The figure shows three views and two pictorial views of one solid part (mm, origin at its lowest corner). Answer the questions. A direction names the side the tool comes from. Round coordinates to 2 decimals unless told otherwise and drop trailing zeros. Order: outer loops, then holes, each group sorted by start corner. A loop starts at its lowest first (then second) coordinate and runs counter-clockwise, first axis right, second up. Notation, with made-up numbers: (58, -15) -> (101, -15) arc R19 ccw to (101, -4) -> close; hole circle Ø5 at (37, -10.5). An arc over 180 degrees is marked (long way). Answer in a Markdown table with one row per item. Add a question column.
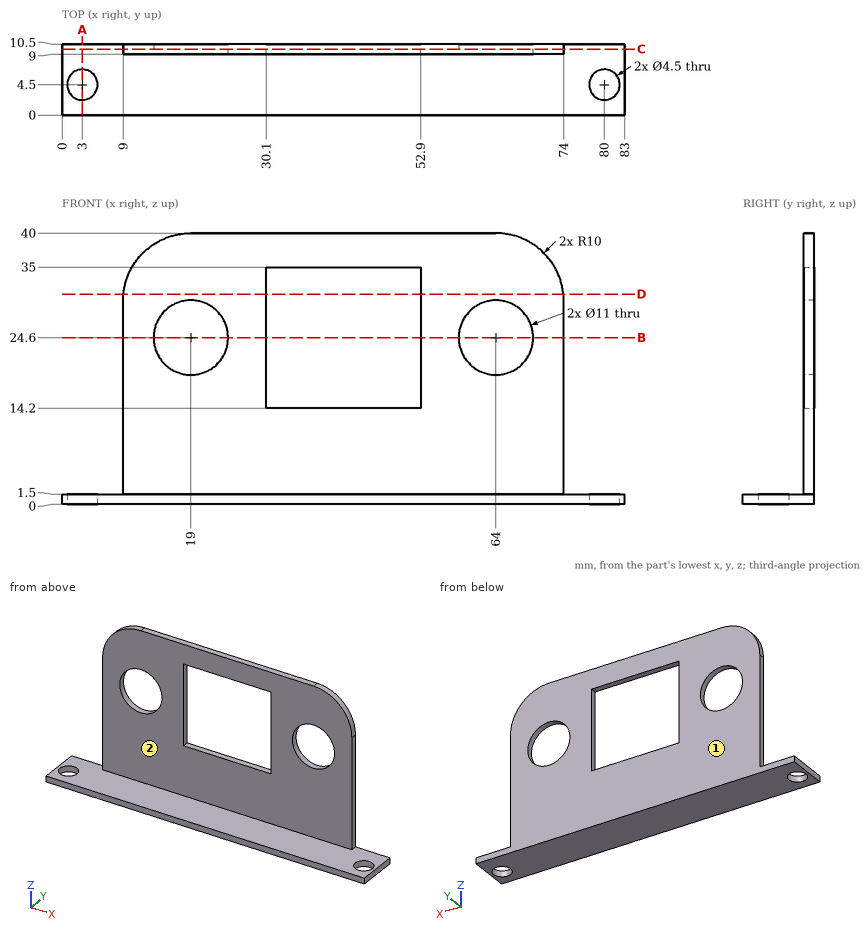
1. The part is cut by section A-A (x = 3). Give the vertices of the cut face in (y, z), then the cut area to 3 significant figures.
2. For the marked faces 1 and 2, determine the directions among +Z, -Z, +X, -X, +Y, -Y from which every point of the face is accessible in a straight line to the end or side of a thin tool.
3. Each of these flat-tipped pins is pushed along its axis until it touches: pin 1 (10 mm diameter, centred on x = 67, z = 13.5, fed in from -Y); pin 2 (2.5 mm diameter, centred on x = 3, y = 4.5, fed in from +Z); pin 3 (0.8 mm diameter, centred on y = 10, z = 20.5, fed in from +X); pin 4 (5 mm diameter, centred on x = 12, y = 3, fed in from +Z). Where does it stop, or does it pass through?
4. Straight lines are drawn through the part: line 1 along Z through (x, y) = (19, 9.4); line 2 along Y through (x, z) = (3, 1.2); line 3 along Y through (x, z) = (32, 3). For each, find the intervals that lie inside material, in ascending order.
5. The part is cut by section C-C (y = 9.75). Give the vertices of the cut face in (x, z).
6. The part is cut by section B-B (z = 24.6). Give the vertices of the cut face in (x, y), then the cut area to 3 significant figures.
7. The part is cut by section D-D (z = 31). Give the vertices of the cut face in (x, y).
Report:
| question | item | result |
|---|---|---|
| 1 | outline | (0, 0) -> (2.25, 0) -> (2.25, 1.5) -> (0, 1.5) -> close; (6.75, 0) -> (10.5, 0) -> (10.5, 1.5) -> (6.75, 1.5) -> close |
| 1 | area | 9.00 mm^2 |
| 2 | face 1 | +Z, -Z, +X, -X, +Y |
| 2 | face 2 | +Z, +X, -X, -Y |
| 3 | pin 1 | stops at y = 9 |
| 3 | pin 2 | passes through |
| 3 | pin 3 | stops at x = 74 |
| 3 | pin 4 | stops at z = 1.5 |
| 4 | line 1 | z = 0 to 19.1, 30.1 to 40 |
| 4 | line 2 | y = 0 to 2.25, 6.75 to 10.5 |
| 4 | line 3 | y = 9 to 10.5 |
| 5 | outline | (0, 0) -> (83, 0) -> (83, 1.5) -> (74, 1.5) -> (74, 30) arc R10 ccw to (64, 40) -> (19, 40) arc R10 ccw to (9, 30) -> (9, 1.5) -> (0, 1.5) -> close; hole circle Ø11 at (19, 24.6); hole (30.1, 14.2) -> (52.9, 14.2) -> (52.9, 35) -> (30.1, 35) -> close; hole circle Ø11 at (64, 24.6) |
| 6 | outline | (9, 9) -> (13.5, 9) -> (13.5, 10.5) -> (9, 10.5) -> close; (24.5, 9) -> (30.1, 9) -> (30.1, 10.5) -> (24.5, 10.5) -> close; (52.9, 9) -> (58.5, 9) -> (58.5, 10.5) -> (52.9, 10.5) -> close; (69.5, 9) -> (74, 9) -> (74, 10.5) -> (69.5, 10.5) -> close |
| 6 | area | 30.3 mm^2 |
| 7 | outline | (9.05, 9) -> (30.1, 9) -> (30.1, 10.5) -> (9.05, 10.5) -> close; (52.9, 9) -> (73.95, 9) -> (73.95, 10.5) -> (52.9, 10.5) -> close |
